from build123d import *

# Parameters (mm, degrees)
F0_W     = 21.91495
F0_H     = 6.17824
F0_W_2   = 23.099592
F0_H_2   = 6.216454
F0_H_3   = 26.751835
F2_DEPTH = 25.4


with BuildPart() as f2:
    # F0 (on Front) → F2 (new body)
    with BuildSketch(Plane.XZ):
        Polygon((-25.084568, 6.17824), (-25.084568, 32.968289), (-46.999518, 35.29929), (-46.999518, 6.17824), align=None)
        Polygon((-3.58351, 32.968289), (-25.084568, 32.968289), (-25.084568, 6.17824), (-25.084568, 0), (-3.58351, 0), (-3.58351, 6.216454), align=None)
        with Locations((-36.042043, 3.08912)):
            Rectangle(F0_W, F0_H)
        with Locations((7.966286, 3.108227)):
            Rectangle(F0_W_2, F0_H_2)
        with Locations((7.966286, 19.592371)):
            Rectangle(F0_W_2, F0_H_3)
    extrude(amount=F2_DEPTH)


solid = f2.part
Source: CAD feature listing. Evaluate the final solid. Frame: model axes, mm. A direction names the side the tool comes from. Give positions to 0.01 mm unless a question says otherwise; leave off trailing zeros. Order: outer loops, then holes, each group sorted by start corner. A loop starts at its lowest first (then second) coordinate and runs counter-clockwise, first axis right, second up. Notation, with made-up numbers: (62.5, -15) -> (73.5, -15) arc R23 cw to (73.5, -6) -> close; hole circle Ø3 at (66, -12). An arc over 180 degrees is marked (long way). Write item = value, one per line.
Item 1: Section query B-B (x = 15.5). Output: boundary loops of the cut face in (y, z), then the cut area to 3 significant figures.
Check result:
outline = (-25.4, 0) -> (0, 0) -> (0, 32.97) -> (-25.4, 32.97) -> close
area = 837 mm²
Item 2: Ray query, probe 1 along Z at (x, y) = (-6.5, -15); probe 2 along Z at (x, y) = (-32.5, -17.25). Return the intervals inside material, ascending.
Check result:
probe_1 = 0 to 32.97
probe_2 = 0 to 33.76
Item 3: Set-up query: faces 4 (the face through (-14, -13, 32.968)), 5 (the face through (19.516, -13, 16)). Return all of +Z, -Z, +X, -X, +Y, -Y with unobstructed straight access to the full face (end or side cutting, diameter ignored); none if empty.
Check result:
face_4 = +Z, +X, +Y, -Y
face_5 = +Z, -Z, +X, +Y, -Y
Item 4: Contact query for a flat-ended pin moving along its axis: pin 1 (1 mm diameter, centred on x = -5.5, y = -19.5, fed in from +Z). Output: stop coordinate, or through.
Check result:
pin_1 = 32.97
Item 5: Section query C-C (x = -30.5). Output: boundary loops of the cut face in (y, z).
Check result:
outline = (-25.4, 0) -> (0, 0) -> (0, 33.54) -> (-25.4, 33.54) -> close
Item 6: Section query A-A (y = -20.75). Output: boundary loops of the cut face in (x, z).
Check result:
outline = (-47, 0) -> (19.52, 0) -> (19.52, 32.97) -> (-25.08, 32.97) -> (-47, 35.3) -> close
Item 7: Mould query, pull axis Z, two halves, no side actions, for faces 1 (the face through (8, -13, 32.968)), 2 (the face through (-14, -25.4, 18)), 3 (the face through (-14, -13, 0)). Classes: +Z half, -Z half, draft (parallel to the pull), parting line (faces both ways), or undercut.
Check result:
face_1 = +Z half
face_2 = draft
face_3 = -Z half
